Input: dimensioned drawing with shaded views. Units: mm. Origin: part minimum x, y, z. A direction names the side the tool comes from. Round coordinates to 2 decimals unless told otherwise and drop trailing zeros. Loops run counter-clockwise (first coordinate to the right, second up) from the corner with the lowest first, then second, coordinate; pieces in that order, holes last. Notation, with made-up numbers: M 85.5,-18.75 L 128.5,-18.75 A21 ccw 128.5,-7.75 Z; hole C 49.25,-9 d5. An arc over 180 degrees is marked long. Return JSON: item names as keys, results as strings.
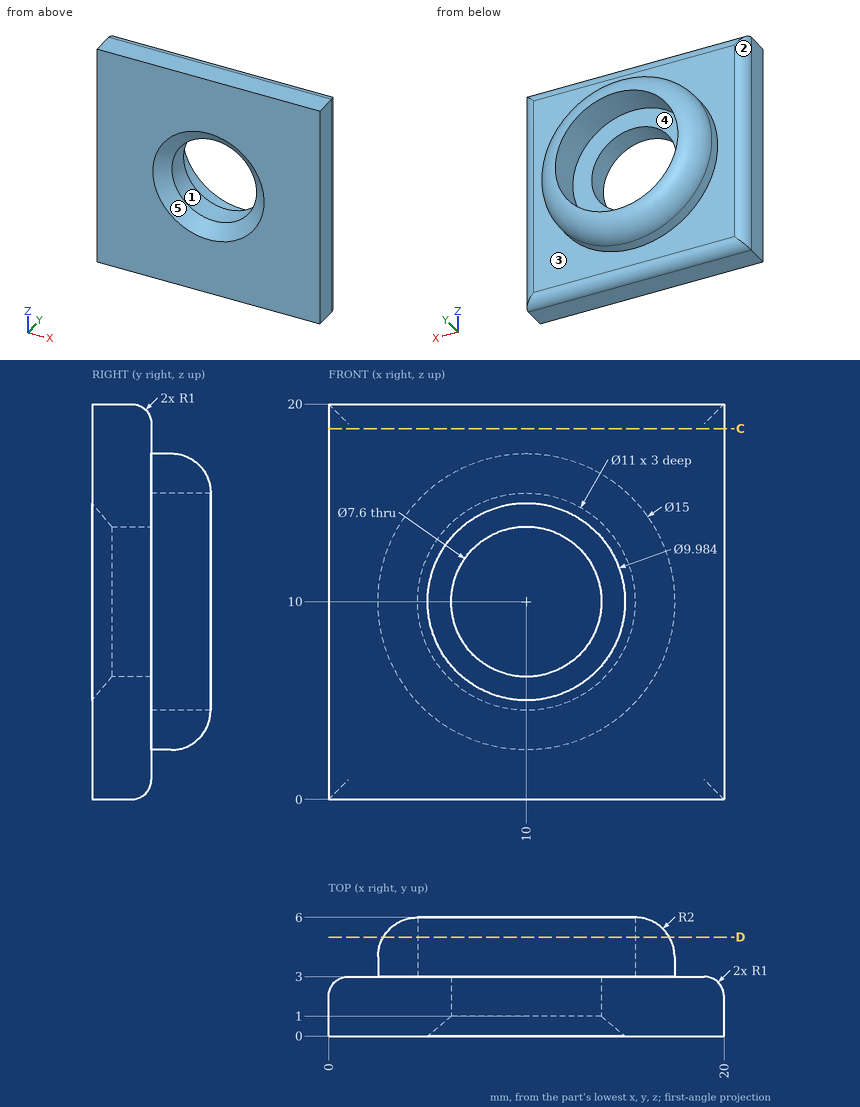
Q1. Pull-direction query (X, two-part tool) for the marked faces 1, 2 and 3; classes: pulls with the +X half, pulls with the -X half, needs draft (parallel to the pull), parting line crosses it, or undercut.
Determined:
{"face 1": "undercut", "face 2": "pulls with the -X half", "face 3": "needs draft"}
Q2. Section query C-C (z = 18.75). Output: boundary loops of the cut face in (x, y).
Determined:
{"outline": "M 0,0 L 20,0 L 20,2 A1 ccw 19,3 L 1,3 A1 ccw 0,2 Z"}
Q3. Pin query (flat end, axial travel): pin 1 (9 mm diameter, centred on x = 10, z = 10, fed in from +Y); pin 2 (1.5 mm diameter, centred on y = 5, z = 8.5, fed in from -X) (1 decimal); pin 3 (9 mm diameter, centred on x = 8.5, z = 12, fed in from +Y); pin 4 (5.5 mm diameter, centred on x = 10.5, z = 9.5, fed in from +Y). Return the tip coordinate at first contact, or that it passes through.
Determined:
{"pin 1": "stops at y = 3", "pin 2": "stops at x = 2.6", "pin 3": "stops at y = 6", "pin 4": "passes through"}
Q4. Reachability of the marked faces 4 and 5 from +Z, -Z, +X, -X, +Y, -Y: full face, straight path, thin tool, end or side. Return the list, or none.
Determined:
{"face 4": "+Y", "face 5": "-Y"}
Q5. Section query D-D (y = 5). Output: boundary loops of the cut face in (x, z) (1 decimal).
Determined:
{"outline": "C 10,10 d14.5; hole C 10,10 d11"}
Q6. Material intervals for L1, parallel to X at y = 1.75, z = 10; L2, parallel to X at y = 3.7, z = 10; L3, parallel to Y at x = 2.5, z = 17.25, sorted ascending.
Determined:
{"L1": "x = 0 to 6.2, 13.8 to 20", "L2": "x = 2.5 to 4.5, 15.5 to 17.5", "L3": "y = 0 to 3"}
